Check sheet for the modelled part. Datum: model origin and axes. Units: mm. Face numbers are marked on the shaded views. A direction names the side the tool comes from. Round coordinates to 2 decimals unless told otherwise and drop trailing zeros. Write each loop counter-clockwise with the first axis right and the second up, starting at its lowest first coordinate (ties: lowest second). Pieces come first, ordered by that corner, then holes.
Item 1: Section check C-C, the plane x = 0. Record the cut outline in (y, z), plus the area to 3 significant figures.
Item 2: Section check A-A, the plane z = 0. Record the cut outline in (x, y).
Item 3: Set-up check for the marked faces 1 and 2: record each of +Z, -Z, +X, -X, +Y, -Y from which the full face is reachable in a straight line by a thin tool's end or side.
Item 4: Section check B-B, the plane y = -25.5. Record the cut outline in (x, z).
Item 5: Section check D-D, the plane z = -4. Record the cut outline in (x, y) (3 decimals).
Item 6: Depth check by flat-ended pin: pin 1 (7.5 mm diameter, centred on y = 6.5, z = -1.5, fed in from +X). Enter the tip coordinate at first touch or a pass-through.
Item 7: Material ranges on line 1 along X through (y, z) = (-19, 0); line 2 along Y through (x, z) = (-7.5, 16.5); line 3 along X through (y, z) = (8.5, -5), recorded low to high.
Item 8: Release check for a two-part mould opening along Z. For the marked faces 3, 4, 5 and 6 record: pulls with the +Z half, pulls with the -Z half, needs draft (parallel to the pull), parting line crosses it, or undercut.
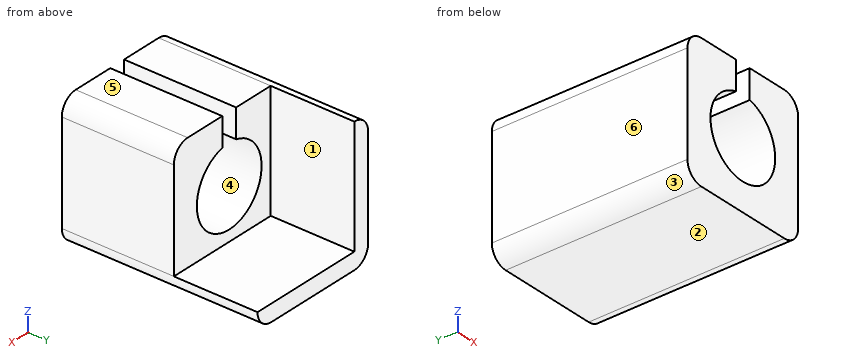
from build123d import *

# Parameters (mm, degrees)
F0_W      = 40
F0_H      = 40
F0_R      = 11.7
F1_DEPTH  = 3.5
F2_R      = 16.7
F2_R_2    = 11.7
F3_DEPTH  = 30
F4_W      = 5
F4_H      = 29.243415
F5_DEPTH  = 33.5
F6_W      = 40
F6_H      = 40
F6_R      = 16.7
F7_DEPTH  = 30.5
F9_DEPTH  = 37.3
F11_DEPTH = 25
F12_R     = 5


with BuildPart() as f1:
    # F0 (on Front) → F1 (new body)
    with BuildSketch(Plane.XZ):
        Rectangle(F0_W, F0_H)
        Circle(F0_R, mode=Mode.SUBTRACT)
    extrude(amount=F1_DEPTH)

    # F2 (on face) → F3 (join)
    with BuildSketch(Plane.XZ.offset(3.5)):
        Circle(F2_R)
        Circle(F2_R_2, mode=Mode.SUBTRACT)
    extrude(amount=F3_DEPTH)

    # F4 (on face) → F5 (cut, through all)
    with BuildSketch(Plane.XZ.offset(33.5)):
        with Locations((0, 14.621707)):
            Rectangle(F4_W, F4_H)
    extrude(amount=-F5_DEPTH, mode=Mode.SUBTRACT)

    # F6 (on face) → F7 (join)
    with BuildSketch(Plane.XZ.offset(33.5)):
        Rectangle(F6_W, F6_H)
        Circle(F6_R, mode=Mode.SUBTRACT)
    extrude(amount=-F7_DEPTH)

    # F8 (on face) → F9 (cut)
    with BuildSketch(Plane.XZ.offset(33.5)):
        Polygon((2.5, 7.926429), (2.5, 11.429786), (2.5, 21.552972), (-2.5, 21.552972), (-2.5, 7.926429), align=None)
    extrude(amount=-F9_DEPTH, mode=Mode.SUBTRACT)

    # F10 (on face) → F11 (join)
    with BuildSketch(Plane(origin=(0, 0, 0), x_dir=(-1, 0, 0), z_dir=(0, 1, 0))):
        Polygon((20, -20), (20, 20), (15, 20), (15, -15), (-20, -15), (-20, -20), align=None)
    extrude(amount=F11_DEPTH)

    # F12
    f12_edges = [f1.edges().sort_by_distance(p)[0] for p in [
        (-20, -4.25, -20),
        (-20, -4.25, 20),
        (20, -4.25, -20),
        (20, -16.75, 20),
    ]]
    fillet(f12_edges, radius=F12_R)


solid = f1.part
Values found:
1. outline: (-33.5, -20) - (25, -20) - (25, -15) - (0, -15) - (0, -11.7) - (-33.5, -11.7) - close
1. area: 403 mm2
2. outline: (-20, -33.5) - (-11.7, -33.5) - (-11.7, 0) - (-15, 0) - (-15, 25) - (-20, 25) - close; (11.7, -33.5) - (20, -33.5) - (20, 0) - (11.7, 0) - close
3. face 1: +Z, +X, +Y
3. face 2: -Z, +X, -X, +Y, -Y
4. outline: (-20, -15) arc R5 ccw to (-15, -20) - (15, -20) arc R5 ccw to (20, -15) - (20, 15) arc R5 ccw to (15, 20) - (2.5, 20) - (2.5, 11.43) arc R11.7 cw (long way) to (-2.5, 11.43) - (-2.5, 20) - (-15, 20) arc R5 ccw to (-20, 15) - close
5. outline: (-20, -33.5) - (-10.995, -33.5) - (-10.995, 0) - (-15, 0) - (-15, 25) - (-20, 25) - close; (10.995, -33.5) - (20, -33.5) - (20, 0) - (10.995, 0) - close
6. pin 1: stops at x = -15
7. line 1: x = -20 to -11.7, 11.7 to 20
7. line 2: y = -33.5 to 0
7. line 3: x = -20 to -15
8. face 3: pulls with the -Z half
8. face 4: undercut
8. face 5: pulls with the +Z half
8. face 6: needs draft
